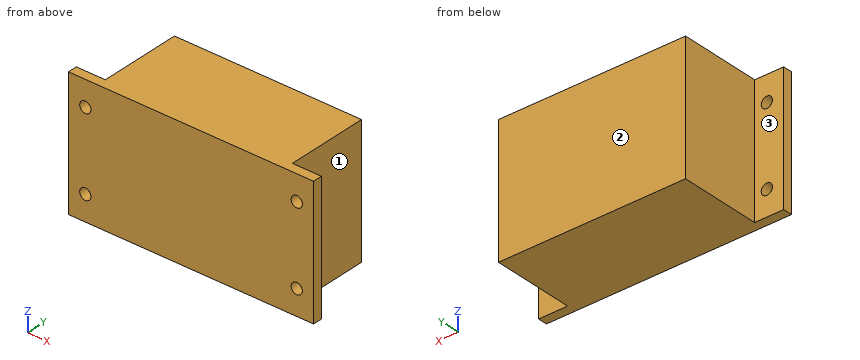
from build123d import *

# Parameters (mm, degrees)
SKETCH_1_W        = 15.5
SKETCH_1_H        = 69
SKETCH_1_R        = 3
EXTRUDE_1_DEPTH   = 5
EXTRUDE_1_2_DEPTH = 5
SKETCH_1_3_W      = 100
SKETCH_1_3_H      = 69
EXTRUDE_2_DEPTH   = 49


with BuildPart() as part:
    # Sketch 1 → Extrude 1 (new body)
    with BuildSketch(Plane(origin=(0, 0, 0), x_dir=(1, 0, 0), z_dir=(0, 1, 0))):
        with Locations((-57.75, 0)):
            Rectangle(SKETCH_1_W, SKETCH_1_H)
        with Locations(Location((-56.5, -21, 0), (0, 0, 270))):
            Circle(SKETCH_1_R, mode=Mode.SUBTRACT)
        with Locations(Location((-56.5, 21, 0), (0, 0, 270))):
            Circle(SKETCH_1_R, mode=Mode.SUBTRACT)
    extrude(amount=EXTRUDE_1_DEPTH)



with BuildPart() as body_2:
    # Sketch 1 → Extrude 1 2 (new body)
    with BuildSketch(Plane(origin=(0, 0, 0), x_dir=(1, 0, 0), z_dir=(0, 1, 0))):
        with Locations((57.75, 0)):
            Rectangle(SKETCH_1_W, SKETCH_1_H)
        with Locations(Location((56.5, -21, 0), (0, 0, 270))):
            Circle(SKETCH_1_R, mode=Mode.SUBTRACT)
        with Locations(Location((56.5, 21, 0), (0, 0, 270))):
            Circle(SKETCH_1_R, mode=Mode.SUBTRACT)
    extrude(amount=EXTRUDE_1_2_DEPTH)


with BuildPart() as part_1:
    add(part.part)

    add(body_2.part)  # Extrude 2 merges body 2
    # Sketch 1_3 → Extrude 2 (add)
    with BuildSketch(Plane(origin=(0, 0, 0), x_dir=(1, 0, 0), z_dir=(0, 1, 0))):
        Rectangle(SKETCH_1_3_W, SKETCH_1_3_H)
    extrude(amount=EXTRUDE_2_DEPTH)


solid = part_1.part
Read the model definition and answer for the solid it produces. Units are mm, in the model's axes. Face numbers are marked on the shaded views. A direction names the side the tool comes from. Round coordinates to 2 decimals unless told otherwise and drop trailing zeros. Order: outer loops, then holes, each group sorted by start corner. A loop starts at its lowest first (then second) coordinate and runs counter-clockwise, first axis right, second up.
1) The part is cut by section A-A on z = 21. Write down the section's boundary in (x, y).
2) The part is cut by section C-C on z = 30. Write down the section's boundary in (x, y).
3) The part is cut by section B-B on x = -56.5. Write down the section's boundary in (y, z), plus the area to 3 significant figures.
4) For the marked faces 1, 2 and 3, determine the directions among +Z, -Z, +X, -X, +Y, -Y from which every point of the face is accessible in a straight line to the end or side of a thin tool.
5) The part is cut by section D-D on y = 23. Write down the section's boundary in (x, z).
6) Straight lines are drawn through the part: L1, parallel to X at y = 3.8, z = -21; L2, parallel to X at y = 44.5, z = -4; L3, parallel to Y at x = -52, z = -16.5. For each, find the intervals that lie inside material, in ascending order.
7) Flat-ended cylindrical pins translate along their axes: pin 1 (4.5 mm diameter, centred on x = 59, z = -16, fed in from +Y); pin 2 (9.5 mm diameter, centred on x = -56.5, z = 21, fed in from -Y); pin 3 (22 mm diameter, centred on y = 32.5, z = 4.5, fed in from +X). Find the tip coordinate at first contact, or state that the pin passes through.
Resolved:
1. outline: (-65.5, 0) - (-59.5, 0) - (-59.5, 5) - (-65.5, 5) - close; (-53.5, 0) - (53.5, 0) - (53.5, 5) - (50, 5) - (50, 49) - (-50, 49) - (-50, 5) - (-53.5, 5) - close; (59.5, 0) - (65.5, 0) - (65.5, 5) - (59.5, 5) - close
2. outline: (-65.5, 0) - (65.5, 0) - (65.5, 5) - (50, 5) - (50, 49) - (-50, 49) - (-50, 5) - (-65.5, 5) - close
3. outline: (0, -34.5) - (5, -34.5) - (5, -24) - (0, -24) - close; (0, -18) - (5, -18) - (5, 18) - (0, 18) - close; (0, 24) - (5, 24) - (5, 34.5) - (0, 34.5) - close
3. area: 285 mm2
4. face 1: +Z, -Z, +X, +Y
4. face 2: +Z, -Z, +X, -X, +Y
4. face 3: +Z, -Z, -X, +Y
5. outline: (-50, -34.5) - (50, -34.5) - (50, 34.5) - (-50, 34.5) - close
6. L1: x = -65.5 to -59.5, -53.5 to 53.5, 59.5 to 65.5
6. L2: x = -50 to 50
6. L3: y = 0 to 5
7. pin 1: stops at y = 5
7. pin 2: stops at y = 0
7. pin 3: stops at x = 50
